```python
from build123d import *

# Parameters (mm, degrees)
SKETCH_1_R                         = 60
EXTRUDE_1_DEPTH                    = 150
CUT_EXTRUDE_START                  = -145
CUT_EXTRUDE_1_DEPTH                = 145
M3X0_5_6MM_D                       = 2.5
CUT_EXTRUDE_START_2                = -22
CUT_EXTRUDE_2_DEPTH                = 22
M3X0_5_SPACER_HUB_BOARD_AT_2_COUNT = 2
M3X0_5_SPACER_HUB_BOARD_AT_2_PITCH = 63.245553203
CUT_EXTRUDE_5070_DEPTH             = 169.002976164
SKETCH_14_R                        = 15
CUT_EXTRUDE_5330_DEPTH             = 173.336879396
M3X0_5_6MM_OBC_D                   = 2.5
FILLET_1_R                         = 1
M5X0_8_20MM_BASW_PLATE_D           = 4.2
M5X0_8_20MM_BASW_PLATE_DEPTH       = 14
M5X0_8_20MM_BASW_PLATE_TIP         = 1.2618073
FILLET_2_R                         = 6
FILLET_3_R                         = 6
SKETCH_19_W                        = 35
SKETCH_19_H                        = 15
CUT_EXTRUDE_3_DEPTH                = 48
FILLET_4_R                         = 7.5
M3X0_5_2_D                         = 2.5
M3X0_5_3_D                         = 2.5


with BuildPart() as part:
    # ｽｹｯﾁ1 → ﾎﾞｽ - 押し出し1 (new body)
    with BuildSketch(Plane(origin=(0, 0, 0), x_dir=(1, 0, 0), z_dir=(0, 1, 0))):
        with Locations(Location((0, 0, 0), (0, 0, 270))):
            Circle(SKETCH_1_R)
    extrude(amount=EXTRUDE_1_DEPTH)

    # ｽｹｯﾁ2 → ｶｯﾄ - 押し出し1 (cut)
    with BuildSketch(Plane(origin=(0, 150, 0), x_dir=(1, 0, 0), z_dir=(0, 1, 0)).offset(CUT_EXTRUDE_START)):
        with BuildLine():
            Line((-44.72135955, 40), (-9.72135955, 40))
            Line((-9.72135955, 40), (-9.72135955, -40))
            Line((-9.72135955, -40), (-44.72135955, -40))
            ThreePointArc((-44.72135955, -40), (-60, 0), (-44.72135955, 40))
        make_face()
    cut_extrude_1 = extrude(amount=CUT_EXTRUDE_1_DEPTH, mode=Mode.SUBTRACT)

    # ﾐﾗｰ1: ｶｯﾄ - 押し出し1 across plane
    add(cut_extrude_1.mirror(Plane(origin=(0, 0, 0), x_dir=(0, 0, 1), z_dir=(1, 0, 0))), mode=Mode.SUBTRACT)

    # ｽｹｯﾁ4 → M6x1.0(20mm) Base_Plateへの固定用ねじ穴 (revolve, cut)
    with BuildSketch(Plane(origin=(0, 0, 30), x_dir=(0, 0, -1), z_dir=(1, 0, 0))):
        Polygon((0, 0), (0, 18.502151548), (2.5, 17), (2.5, 0), align=None)
    m6x1_0_20mm_base_plate = revolve(axis=Axis((0, -6.35, 30), (0, 1, 0)), mode=Mode.SUBTRACT)

    # ﾐﾗｰ2: M6x1.0(20mm) Base_Plateへの固定用ねじ穴 across plane
    add(m6x1_0_20mm_base_plate.mirror(Plane.XY), mode=Mode.SUBTRACT)

    # M3x0.5(6mm) 送信機固定用ねじ穴 (through all)
    with Locations(Plane(origin=(9.72135955, 144, 17.5), x_dir=(0, 0, 1), z_dir=(1, 0, 0))):
        with Locations((0, 0), (-17.5, 0), (-35, 0), (-17.5, 114), (0, 114), (-35, 114)):
            Hole(M3X0_5_6MM_D / 2)

    # ｽｹｯﾁ10 → ｶｯﾄ - 押し出し2 (cut)
    with BuildSketch(Plane(origin=(0, 150, 0), x_dir=(1, 0, 0), z_dir=(0, 1, 0)).offset(CUT_EXTRUDE_START_2)):
        with BuildLine():
            Line((-30, 40), (-44.72135955, 40))
            ThreePointArc((-44.72135955, 40), (0, 60), (44.72135955, 40))
            Line((44.72135955, 40), (30, 40))
            ThreePointArc((30, 40), (0, 50), (-30, 40))
        make_face()
    cut_extrude_2 = extrude(amount=CUT_EXTRUDE_2_DEPTH, mode=Mode.SUBTRACT)

    # ﾐﾗｰ3: ｶｯﾄ - 押し出し2 across plane
    add(cut_extrude_2.mirror(Plane.XY), mode=Mode.SUBTRACT)

    # ｽｹｯﾁ12 → M3x0.5(Spacer) Hub_Board固定用ねじ穴 (revolve, cut)
    with BuildSketch(Plane(origin=(-31.622776602, 128, -45), x_dir=(0, 0, 1), z_dir=(1, 0, 0))):
        Polygon((0, 0), (0, 9.251075774), (1.25, 8.5), (1.25, 0), align=None)
    m3x0_5_spacer_hub_board = revolve(axis=Axis((-31.622776602, 134.35, -45), (0, -1, 0)), mode=Mode.SUBTRACT)

    # M3x0.5(Spacer) Hub_Board固定用ねじ穴 at 2: M3x0.5(Spacer) Hub_Board固定用ねじ穴 ×2
    with Locations(*[(i * M3X0_5_SPACER_HUB_BOARD_AT_2_PITCH, 0, 0) for i in range(1, M3X0_5_SPACER_HUB_BOARD_AT_2_COUNT)]):
        add(m3x0_5_spacer_hub_board, mode=Mode.SUBTRACT)

    # ﾐﾗｰ4: M3x0.5(Spacer) Hub_Board固定用ねじ穴 across plane
    add(m3x0_5_spacer_hub_board.mirror(Plane.XY), mode=Mode.SUBTRACT)

    # ﾐﾗｰ4 copy 1 sketch → ﾐﾗｰ4 copy 1 (revolve, cut)
    with BuildSketch(Plane(origin=(31.622776602, 128, 45), x_dir=(0, 0, -1), z_dir=(1, 0, 0))):
        Polygon((0, 0), (0, -9.251075774), (1.25, -8.5), (1.25, 0), align=None)
    revolve(axis=Axis((31.622776602, 134.35, 45), (0, 1, 0)), mode=Mode.SUBTRACT)

    # ｽｹｯﾁ13 → Cut-Extrude 5070 (cut, through all)
    with BuildSketch(Plane(origin=(0, 5, 0), x_dir=(1, 0, 0), z_dir=(0, 1, 0))):
        with BuildLine():
            Line((-25, 20), (-56.568542495, 20))
            ThreePointArc((-56.568542495, 20), (-60, 0), (-56.568542495, -20))
            Line((-56.568542495, -20), (-25, -20))
            Line((-25, -20), (-25, 20))
        make_face()
    extrude(amount=-CUT_EXTRUDE_5070_DEPTH, mode=Mode.SUBTRACT)

    # ｽｹｯﾁ14 → Cut-Extrude 5330 (cut, through all)
    with BuildSketch(Plane.XZ):
        with Locations(Location((40, 0, 0), (0, 0, 270))):
            Circle(SKETCH_14_R)
    extrude(amount=-CUT_EXTRUDE_5330_DEPTH, mode=Mode.SUBTRACT)

    # M3x0.5(6mm) OBC固定用ねじ穴 (through all)
    with Locations(Plane(origin=(-9.72135955, 139, -30), x_dir=(0, 0, -1), z_dir=(-1, 0, 0))):
        with Locations((0, 0), (-60, 0), (0, 114), (-60, 114)):
            Hole(M3X0_5_6MM_OBC_D / 2)

    # ﾌｨﾚｯﾄ1
    fillet_1_edges = [part.edges().sort_by_distance(p)[0] for p in [
        (-25, 2.5, -20),
        (-25, 2.5, 20),
    ]]
    fillet(fillet_1_edges, radius=FILLET_1_R)

    # M5x0.8(20mm) Basw_Plateへの固定用ねじ穴
    with Locations(Plane(origin=(-25, 0, 46.733285782), x_dir=(0, 0, -1), z_dir=(0, -1, 0))):
        with Locations((0, 0), (0, 50), (93.466571564, 0), (93.466571564, 50)):
            Hole(M5X0_8_20MM_BASW_PLATE_D / 2, depth=M5X0_8_20MM_BASW_PLATE_DEPTH)
            with Locations((0, 0, -(M5X0_8_20MM_BASW_PLATE_DEPTH + M5X0_8_20MM_BASW_PLATE_TIP / 2))):  # 118° drill point
                Cone(0, M5X0_8_20MM_BASW_PLATE_D / 2, M5X0_8_20MM_BASW_PLATE_TIP, mode=Mode.SUBTRACT)

    # ﾌｨﾚｯﾄ2
    fillet_2_edges = [part.edges().sort_by_distance(p)[0] for p in [
        (27.22135955, 5, 40),
        (27.22135955, 5, -40),
    ]]
    fillet(fillet_2_edges, radius=FILLET_2_R)

    # ﾌｨﾚｯﾄ3
    fillet_3_edges = [part.edges().sort_by_distance(p)[0] for p in [
        (-27.22135955, 5, -40),
        (-27.22135955, 5, 40),
    ]]
    fillet(fillet_3_edges, radius=FILLET_3_R)

    # ｽｹｯﾁ19 → ｶｯﾄ - 押し出し3 (cut)
    with BuildSketch(Plane(origin=(9.72135955, 0, 0), x_dir=(0, 0, -1), z_dir=(1, 0, 0))):
        with Locations((0, 17.5)):
            Rectangle(SKETCH_19_W, SKETCH_19_H)
    extrude(amount=-CUT_EXTRUDE_3_DEPTH, mode=Mode.SUBTRACT)

    # ﾌｨﾚｯﾄ4
    fillet_4_edges = [part.edges().sort_by_distance(p)[0] for p in [
        (0, 25, 17.5),
        (0, 10, 17.5),
        (0, 10, -17.5),
        (0, 25, -17.5),
    ]]
    fillet(fillet_4_edges, radius=FILLET_4_R - 0.0001)  # a hair under: the kernel refuses the full size

    # M3x0.5 ねじ穴2 (through all)
    with Locations(Plane(origin=(-45, 5, -25), x_dir=(0, 0, 1), z_dir=(0, 1, 0))):
        with Locations((0, 0), (0, 20), (50, 20), (50, 0)):
            Hole(M3X0_5_2_D / 2)

    # M3x0.5 ねじ穴3 (through all)
    with Locations(Plane(origin=(9.72135955, 127, 30), x_dir=(0, 0, 1), z_dir=(1, 0, 0))):
        with Locations((0, 0), (0, 80), (-60, 80), (-60, 0)):
            Hole(M3X0_5_3_D / 2)


solid = part.part
```
Verification items for the finished model (mm, model axes). A direction names the side the tool comes from. Give positions to 0.01 mm unless a question says otherwise; leave off trailing zeros. Write each loop counter-clockwise with the first axis right and the second up, starting at its lowest first coordinate (ties: lowest second). Pieces come first, ordered by that corner, then holes. Notation, with made-up numbers: (41.25, 84.25) - (63.25, 84.25) arc R23 cw to (63.25, 120.25) - close; hole circle Ø5 at (85.5, -34.5). An arc over 180 degrees is marked (long way). Put each result on its own line as item: value.
Q1. Set-up check for faces 1 (the face through (23, 5, 0)), 2 (the face through (-0.1, 8.4, -32.5)), 3 (the face through (-9.721, 76, -1)): record each of +Z, -Z, +X, -X, +Y, -Y from which the full face is reachable in a straight line by a thin tool's end or side.
Result:
face 1: +X, +Y
face 2: -Y
face 3: -X, +Y
Q2. Section check B-B on y = 60.5. Record the cut outline in (x, z), and give its area (3 significant figures).
Result:
outline: (-44.72, -40) arc R60 ccw to (44.72, -40) - (9.72, -40) - (9.72, 40) - (44.72, 40) arc R60 ccw to (-44.72, 40) - (-9.72, 40) - (-9.72, -40) - close
area: 4,030 mm2
Q3. Depth check by flat-ended pin: P1, Ø3, axis at y = 144, z = 17.5, coming from the -X side; P2, Ø9.5, axis at x = 0.5, z = 4, coming from the -Y side; P3, Ø4.5, axis at x = 0, z = 30, coming from the -Y side; P4, Ø6, axis at y = 80, z = 45, coming from the -X side. Enter the tip coordinate at first touch or a pass-through.
Result:
P1: x = -9.72
P2: y = 0
P3: y = 17.15
P4: x = -42.85
Q4. Mould release check, pull along X, two halves, no side actions. Record for faces 4 (the face through (0, 139, 50)), 5 (the face through (0.17, 18.24, 29.6)), 6 (the face through (-22, 5, 0)): released by +X, released by -X, zero draft, split by the parting line, or undercut.
Result:
face 4: split by the parting line
face 5: undercut
face 6: zero draft
Q5. Section check D-D on y = 133. Record the cut outline in (x, z).
Result:
outline: (-30, -40) arc R50 ccw to (30, -40) - (9.72, -40) - (9.72, 40) - (30, 40) arc R50 ccw to (-30, 40) - (-9.72, 40) - (-9.72, -40) - close
Q6. Section check C-C on x = 12. Record the cut outline in (y, z), and give its area (3 significant figures).
Result:
outline: (0, -58.79) - (128, -58.79) - (128, -48.54) - (150, -48.54) - (150, -40) - (11, -40) arc R6 cw to (5, -34) - (5, 34) arc R6 cw to (11, 40) - (150, 40) - (150, 48.54) - (128, 48.54) - (128, 58.79) - (0, 58.79) - close
area: 5,600 mm2
Q7. Scan lines: probe 1 along Z at (x, y) = (0, 9); probe 2 along Z at (x, y) = (0, 139); probe 3 along Y at (x, z) = (1, 0). Record each from-to range of solid material in increasing order. Write a range as from..to.
Result:
probe 1: -60..-32.5, -27.5..27.5, 32.5..60
probe 2: -50..-31.25, -28.75..28.75, 31.25..50
probe 3: 0..10, 25..28.75, 31.25..142.75, 145.25..150
Q8. Section check A-A on x = -41. Record the cut outline in (y, z).
Result:
outline: (0, -43.81) - (128, -43.81) - (128, -40) - (11, -40) arc R6 cw to (5, -34) - (5, -20) - (0, -20) - close; (0, 20) - (5, 20) - (5, 34) arc R6 cw to (11, 40) - (128, 40) - (128, 43.81) - (0, 43.81) - close
